Read the model definition and answer for the solid it produces. Units are mm, in the model's axes. Face numbers are marked on the shaded views. A direction names the side the tool comes from. Round coordinates to 2 decimals unless told otherwise and drop trailing zeros. Loops run counter-clockwise (first coordinate to the right, second up) from the corner with the lowest first, then second, coordinate; pieces in that order, holes last. Notation, with made-up numbers: M -37.75,24 L 1.25,24 A33 cw 1.25,60 Z; hole C 30,-29 d2. An arc over 180 degrees is marked long. Write each question's results on one line, items separated by ' | '.
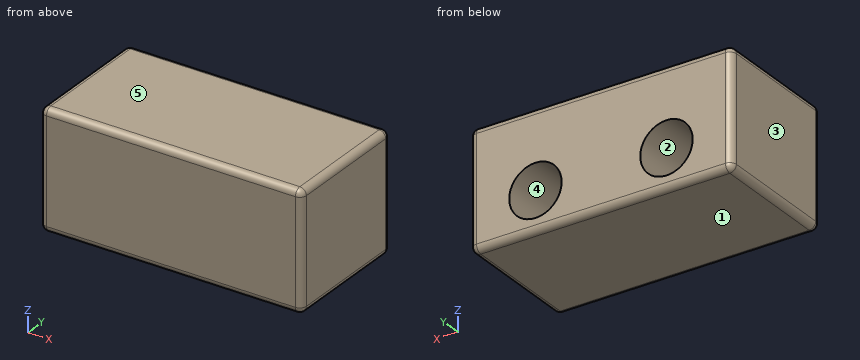
```python
from build123d import *

# Parameters (mm, degrees)
BOSS_EXTRUDE1_DEPTH = 10
SKETCH2_R           = 2
CUT_EXTRUDE1_DEPTH  = 5
FILLET2_R           = 0.5


with BuildPart() as part:
    # Sketch1 → Boss-Extrude1 (new body)
    with BuildSketch(Plane(origin=(0, 0, 0), x_dir=(1, 0, 0), z_dir=(0, 1, 0))):
        Polygon((-9.137931034, 3.146551724), (10.862068966, 3.146551724), (10.862068966, -1.853448276), (10.862068966, -5.853448276), (-9.137931034, -5.853448276), (-9.137931034, -1.853448276), align=None)
    extrude(amount=BOSS_EXTRUDE1_DEPTH)

    # Sketch2 → Cut-Extrude1 (cut)
    with BuildSketch(Plane(origin=(0, 10, 0), x_dir=(1, 0, 0), z_dir=(0, 1, 0))):
        with Locations(Location((-4.137931034, 0.146551724, 0), (0, 0, 270))):
            Circle(SKETCH2_R)
        with Locations(Location((5.862068966, 0.146551724, 0), (0, 0, 270))):
            Circle(SKETCH2_R)
    extrude(amount=-CUT_EXTRUDE1_DEPTH, mode=Mode.SUBTRACT)

    # Fillet2
    fillet2_edges = [part.edges().sort_by_distance(p)[0] for p in [
        (-9.137931034, 5, -3.146551724),
        (10.862068966, 5, -3.146551724),
        (10.862068966, 5, 5.853448276),
        (-9.137931034, 5, 5.853448276),
        (0.862068966, 10, 5.853448276),
        (10.862068966, 10, 1.353448276),
        (0.862068966, 10, -3.146551724),
        (-9.137931034, 10, 1.353448276),
        (0.862068966, 0, -3.146551724),
        (10.862068966, 0, 1.353448276),
        (0.862068966, 0, 5.853448276),
        (-9.137931034, 0, 1.353448276),
    ]]
    fillet(fillet2_edges, radius=FILLET2_R)


solid = part.part
```
1. Which of the six approach directions +Z, -Z, +X, -X, +Y, -Y give full straight-line access (tool end or side, diameter ignored) to the marked faces 1 and 2?
Completed:
face 1: -Z, +X, -X, +Y, -Y | face 2: +Y
2. Find section B-B, the plane z = -0.25. Give the vertices of the cut face in (x, y), then the cut area to 3 significant figures.
Completed:
outline: M -9.14,0.5 A0.5 ccw -8.64,0 L 10.36,0 A0.5 ccw 10.86,0.5 L 10.86,9.5 A0.5 ccw 10.36,10 L 7.86,10 L 7.86,5 L 3.86,5 L 3.86,10 L -2.14,10 L -2.14,5 L -6.14,5 L -6.14,10 L -8.64,10 A0.5 ccw -9.14,9.5 Z | area: 160 mm2
3. Given P1, Ø3.5, axis at x = -4.14, z = -0.15, coming from the -Y side, flat-ended and moving along its own axis, determine where the tip first touches the part or whether it passes through.
Completed:
P1: stops at y = 0
4. Determine the mould class of the marked faces 3, 4 and 5 for opening direction Z: released by +Z, released by -Z, zero draft, split by the parting line, or undercut.
Completed:
face 3: zero draft | face 4: undercut | face 5: released by +Z
5. Find section C-C, the plane z = -1.75. Give the vertices of the cut face in (x, y).
Completed:
outline: M -9.14,0.5 A0.5 ccw -8.64,0 L 10.36,0 A0.5 ccw 10.86,0.5 L 10.86,9.5 A0.5 ccw 10.36,10 L 7.06,10 L 7.06,5 L 4.67,5 L 4.67,10 L -2.94,10 L -2.94,5 L -5.33,5 L -5.33,10 L -8.64,10 A0.5 ccw -9.14,9.5 Z
6. Find section A-A, the plane y = 8.25. Give the vertices of the cut face in (x, z).
Completed:
outline: M -9.14,-2.65 A0.5 ccw -8.64,-3.15 L 10.36,-3.15 A0.5 ccw 10.86,-2.65 L 10.86,5.35 A0.5 ccw 10.36,5.85 L -8.64,5.85 A0.5 ccw -9.14,5.35 Z; hole C -4.14,-0.15 d4; hole C 5.86,-0.15 d4
7. Find the intervals of material crossed by L1, parallel to X at y = 9, z = -0.25; L2, parallel to Y at x = -3.5, z = -2; L3, parallel to X at y = 8.25, z = -1, in increasing order.
Completed:
L1: x = -9.14 to -6.14, -2.14 to 3.86, 7.86 to 10.86 | L2: y = 0 to 5 | L3: x = -9.14 to -5.95, -2.33 to 4.05, 7.67 to 10.86
